from build123d import *

# Parameters (mm, degrees)
SKETCH1_R               = 6
BOSS_EXTRUDE1_DEPTH     = 3
SKETCH2_R               = 0.75
CUT_EXTRUDE1_DEPTH      = 9.4
CUT_EXTRUDE1_DEPTH_BACK = 4.6


with BuildPart() as part:
    # Sketch1 → Boss-Extrude1 (new body)
    with BuildSketch(Plane(origin=(0, 0, 0), x_dir=(0, 0, -1), z_dir=(1, 0, 0))):
        Circle(SKETCH1_R)
        with BuildLine():
            Line((-3.865553001, 2.4), (3.865553001, 2.4))
            ThreePointArc((3.865553001, 2.4), (4.55, 0), (3.865553001, -2.4))
            Line((3.865553001, -2.4), (-3.865553001, -2.4))
            ThreePointArc((-3.865553001, -2.4), (-4.55, 0), (-3.865553001, 2.4))
        make_face(mode=Mode.SUBTRACT)
    extrude(amount=BOSS_EXTRUDE1_DEPTH)

    # Sketch2 → Cut-Extrude1 (cut, two sides)
    with BuildSketch(Plane(origin=(0, -2.4, 0), x_dir=(1, 0, 0), z_dir=(0, 1, 0))) as cut_extrude1_sk:
        with Locations((1.5, 0)):
            Circle(SKETCH2_R)
    extrude(amount=CUT_EXTRUDE1_DEPTH, mode=Mode.SUBTRACT)
    extrude(cut_extrude1_sk.sketch, amount=-CUT_EXTRUDE1_DEPTH_BACK, mode=Mode.SUBTRACT)


solid = part.part
The listing builds one solid part. Answer for the finished solid, in the listing's coordinates (mm). A direction names the side the tool comes from. Coordinates: 2 decimals unless noted, no trailing zeros. Loops run counter-clockwise (first coordinate to the right, second up) from the corner with the lowest first, then second, coordinate; pieces in that order, holes last.
1) Find section C-C on x = 1.45. Write down the section's boundary in (y, z).
2) Find the intervals of material crossed by L1, parallel to X at y = -4.9, z = 0; L2, parallel to Z at x = 0.8, y = -0.75; L3, parallel to Y at x = 1.2, z = -2.5, in increasing order.
3) Find section A-A on z = 0. Write down the section's boundary in (x, y), then the cut area to 3 significant figures.
4) Determine the mould class of faces 3 (the face through (1, 0, 6)), 4 (the face through (1.48, -0.04, 4.55)), 5 (the face through (2.19, 4.17, 0.29)) for opening direction Y: pulls with the +Y half, pulls with the -Y half, needs draft (parallel to the pull), parting line crosses it, or undercut.
5) A tool of negligible diameter and unlimited length cuts with its end or side. For faces 1 (the face through (2.19, -4.17, 0.29)), 2 (the face through (1, -2.4, -1)), from which of +Z, -Z, +X, -X, +Y, -Y can it reach the whole face along a straight path? Write none if from no direction.
6) Find section B-B on y = 0. Write down the section's boundary in (x, z).
7) Flat-ended cylindrical pins translate along their axes: pin 1 Ø1.5 at (x, z) = (1, -3) entering from -Y; pin 2 Ø1.2 at (x, z) = (1.5, 0) entering from -Y; pin 3 Ø0.9 at (x, z) = (1.5, -0.5) entering from -Y. Find the tip coordinate at first contact, or state that the pin passes through.
8) Find section D-D on z = -1.25. Write down the section's boundary in (x, y), then the cut area to 3 significant figures.
Values:
1. outline: (-5.95, -0.75) arc R6 ccw to (5.95, -0.75) - (2.4, -0.75) - (2.4, -3.87) arc R4.55 cw to (-2.4, -3.87) - (-2.4, -0.75) - close; (-5.95, 0.75) - (-2.4, 0.75) - (-2.4, 3.87) arc R4.55 cw to (2.4, 3.87) - (2.4, 0.75) - (5.95, 0.75) arc R6 ccw to start
2. L1: x = 0 to 0.75, 2.25 to 3
2. L2: z = -5.95 to -4.49, 4.49 to 5.95
2. L3: y = -5.45 to -2.4, 2.4 to 5.45
3. outline: (0, -6) - (0.75, -6) - (0.75, -2.4) - (0, -2.4) - close; (0, 2.4) - (0.75, 2.4) - (0.75, 6) - (0, 6) - close; (2.25, -6) - (3, -6) - (3, -2.4) - (2.25, -2.4) - close; (2.25, 2.4) - (3, 2.4) - (3, 6) - (2.25, 6) - close
3. area: 10.8 mm2
4. face 3: parting line crosses it
4. face 4: undercut
4. face 5: needs draft
5. face 1: +Y, -Y
5. face 2: +X, -X
6. outline: (0, -6) - (3, -6) - (3, -4.55) - (0, -4.55) - close; (0, 4.55) - (3, 4.55) - (3, 6) - (0, 6) - close
7. pin 1: stops at y = -5.56
7. pin 2: passes through
7. pin 3: stops at y = -5.97
8. outline: (0, -5.87) - (3, -5.87) - (3, -2.4) - (0, -2.4) - close; (0, 2.4) - (3, 2.4) - (3, 5.87) - (0, 5.87) - close
8. area: 20.8 mm2
